Design review of the part built by this model. Coordinates are the model's own, in mm. A direction names the side the tool comes from. Give positions to 0.01 mm unless a question says otherwise; leave off trailing zeros. Order: outer loops, then holes, each group sorted by start corner. A loop starts at its lowest first (then second) coordinate and runs counter-clockwise, first axis right, second up. Notation, with made-up numbers: (83, 75.5) -> (119, 75.5) arc R20 cw to (119, 83.5) -> close; hole circle Ø8 at (-5.75, -16.5). An arc over 180 degrees is marked (long way). Use a Markdown table: item, result. Add a question column.
```python
from build123d import *

# Parameters (mm, degrees)
F1_DEPTH = 71.4375
F2_R     = 3.683
F2_R_2   = 2.0193
F3_DEPTH = 9.526
F4_R     = 2.0447
F5_DEPTH = 20.321
F6_W     = 19.05
F6_H     = 23.8125
F7_DEPTH = 3.556


with BuildPart() as f1:
    # F0 (on Front) → F1 (new body)
    with BuildSketch(Plane.XZ):
        Polygon((9.525, 9.525), (-9.525, 9.525), (-9.525, 3.302), (-10.795, 3.302), (-10.795, 0), (-5.715, 0), (-5.715, 5.969), (5.715, 5.969), (5.715, 0), (10.795, 0), (10.795, 3.302), (9.525, 3.302), align=None)
    extrude(amount=F1_DEPTH)

    # F2 (on face) → F3 (cut, through all)
    with BuildSketch(Plane.XY.offset(9.525)):
        with Locations((0, -50.2285)):
            Circle(F2_R)
        with Locations((0, -63.8683)):
            Circle(F2_R_2)
    extrude(amount=-F3_DEPTH, mode=Mode.SUBTRACT)

    # F4 (on face) → F5 (cut, through all)
    with BuildSketch(Plane.YZ.offset(9.525)):
        with Locations((-58.1025, 6.096)):
            Circle(F4_R)
    extrude(amount=-F5_DEPTH, mode=Mode.SUBTRACT)

    # F6 (on face) → F7 (cut)
    with BuildSketch(Plane.XY.offset(9.525)):
        with Locations((0, -26.19375)):
            Rectangle(F6_W, F6_H)
    extrude(amount=-F7_DEPTH, mode=Mode.SUBTRACT)


solid = f1.part
```
1) Add section A-A (x = 0). Give the boundary of the cut face in (y, z) (1 decimal).
2) For L1, parallel to Y at x = 0, z = 7.5; L2, parallel to X at y = -16.5, z = 2 (3 decimals); L3, parallel to X at y = -11.5, z = 3.75 (3 decimals), list the stretches that pass through material, from the lowest coordinate up. Write a range as [from, to].
3) Add section D-D (y = -59.5). Give the boundary of the cut face in (x, z) (3 decimals), then the cut area to 3 significant figures.
4) Machinability: for faces 4 (the flat face through (0, -45, 5.969)), 5 (the flat face through (9.525, -35.2, 5.7)), 6 (the flat face through (0, -38.1, 8)), 7 (the flat face through (-9.525, -35.2, 5.8)), 8 (the flat face through (8, -35, 0)), which of the approach directions +Z, -Z, +X, -X, +Y, -Y give a long, thin tool a straight path to every point of the face, cutting with its end or side? Answer none if there is none.
5) Add section B-B (y = -37). Give the boundary of the cut face in (x, z) (3 decimals).
6) The part is to be moulded in two halves that separate along X. For faces 1 (the flat face through (-10.795, -35, 2)), 2 (the flat face through (-8, -26, 5.969)), 3 (the flat face through (0, -67, 5.969)), say which applies: +X half, -X half, draft (parallel to the pull), parting line (faces both ways), or undercut.
7) Add section C-C (z = 1.75). Give the boundary of the cut face in (x, y) (1 decimal), then the cut area to 3 significant figures.
8) Insertion check: pin 1 (4.5 mm diameter, centred on y = -58.1, z = 6.1, fed in from -X) (3 decimals); pin 2 (3.5 mm diameter, centred on x = -1.5, y = -8.5, fed in from -Z); pin 3 (1.1 mm diameter, centred on x = 8.5, y = -28, fed in from +Z); pin 4 (3.5 mm diameter, centred on x = 0, y = -63.87, fed in from +Z). Each pin has a flat end and moves straight along its axis. Give the tip position at first contact, or say it passes through.
Worked answers:
| question | item | result |
|---|---|---|
| 1 | outline | (-71.4, 6) -> (-65.9, 6) -> (-65.9, 9.5) -> (-71.4, 9.5) -> close; (-61.8, 6) -> (-60.1, 6) arc R2 cw (long way) to (-56.1, 6) -> (-53.9, 6) -> (-53.9, 9.5) -> (-61.8, 9.5) -> close; (-46.5, 6) -> (-38.1, 6) -> (-38.1, 9.5) -> (-46.5, 9.5) -> close; (-14.3, 6) -> (0, 6) -> (0, 9.5) -> (-14.3, 9.5) -> close |
| 2 | L1 | [-71.44, -65.89], [-61.85, -59.59], [-56.62, -53.91], [-46.55, -38.1], [-14.29, 0] |
| 2 | L2 | [-10.795, -5.715], [5.715, 10.795] |
| 2 | L3 | [-9.525, -5.715], [5.715, 9.525] |
| 3 | outline | (-10.795, 0) -> (-5.715, 0) -> (-5.715, 4.603) -> (-9.525, 4.603) -> (-9.525, 3.302) -> (-10.795, 3.302) -> close; (-9.525, 7.589) -> (9.525, 7.589) -> (9.525, 9.525) -> (-9.525, 9.525) -> close; (5.715, 0) -> (10.795, 0) -> (10.795, 3.302) -> (9.525, 3.302) -> (9.525, 4.603) -> (5.715, 4.603) -> close |
| 3 | area | 80.4 mm^2 |
| 4 | face 4 | -Z, +Y, -Y |
| 4 | face 5 | +Z, +X, +Y, -Y |
| 4 | face 6 | +Z, +X, -X |
| 4 | face 7 | +Z, -X, +Y, -Y |
| 4 | face 8 | -Z, +X, -X, +Y, -Y |
| 5 | outline | (-10.795, 0) -> (-5.715, 0) -> (-5.715, 5.969) -> (-9.525, 5.969) -> (-9.525, 3.302) -> (-10.795, 3.302) -> close; (5.715, 0) -> (10.795, 0) -> (10.795, 3.302) -> (9.525, 3.302) -> (9.525, 5.969) -> (5.715, 5.969) -> close |
| 6 | face 1 | -X half |
| 6 | face 2 | draft |
| 6 | face 3 | undercut |
| 7 | outline | (-10.8, -71.4) -> (-5.7, -71.4) -> (-5.7, 0) -> (-10.8, 0) -> close; (5.7, -71.4) -> (10.8, -71.4) -> (10.8, 0) -> (5.7, 0) -> close |
| 7 | area | 726 mm^2 |
| 8 | pin 1 | x = -9.525 |
| 8 | pin 2 | z = 5.97 |
| 8 | pin 3 | z = 5.97 |
| 8 | pin 4 | through |
